Design review of the part built by this model. Coordinates are the model's own, in mm. Give positions to 0.01 mm unless a question says otherwise; leave off trailing zeros. Write each loop counter-clockwise with the first axis right and the second up, starting at its lowest first coordinate (ties: lowest second). Pieces come first, ordered by that corner, then holes. Notation, with made-up numbers: M 60,59.25 L 115,59.25 A18 cw 115,75.25 Z; hole C 79,10 d8. An arc over 180 degrees is marked long. Answer in a Markdown table with one row per item.
```python
from build123d import *

# Parameters (mm, degrees)
F0_R     = 30
F0_R_2   = 9.5
F1_DEPTH = 20
F2_DEPTH = 8
F3_D     = 5.5


with BuildPart() as f1:
    # F0 (on Front) → F1 (new body)
    with BuildSketch(Plane.XZ):
        Circle(F0_R)
        with Locations((17.2907616943, 0)):
            Circle(F0_R_2, mode=Mode.SUBTRACT)
        with Locations((17.2907616943, 0)):
            Circle(F0_R_2)
    extrude(amount=-F1_DEPTH)

    # F0 (on Front) → F2 (join)
    with BuildSketch(Plane.XZ):
        with Locations((17.2907616943, 0)):
            Circle(F0_R_2)
    extrude(amount=F2_DEPTH)

    # F3 (through all)
    with Locations(Plane.XZ):
        with Locations((0, 0)):
            Hole(F3_D / 2)


solid = f1.part
```
1) The part is to be moulded in two halves that separate along Z. For faces 1 (the face through (17, -8, 0)), 2 (the face through (7.8, -3.9, 0.4)), 3 (the face through (0.596, 10.14, -2.685)), say which applies: released by +Z, released by -Z, zero draft, split by the parting line, or undercut.
Geometry says:
| item | result |
|---|---|
| face 1 | zero draft |
| face 2 | split by the parting line |
| face 3 | undercut |
2) To check wall thickness, follow probe 1 along Z at (x, y) = (0, 6); probe 2 along Y at (x, z) = (27, 9); probe 3 along Z at (x, y) = (1.5, 5.25). State the ranges of each line that lie inside material, in increasing order. Write a range as [from, to].
Geometry says:
| item | result |
|---|---|
| probe 1 | [-30, -2.75], [2.75, 30] |
| probe 2 | [0, 20] |
| probe 3 | [-29.96, -2.3], [2.3, 29.96] |
3) Insertion check: P1, Ø6, axis at y = 4, z = 8.5, coming from the -X side; P2, Ø4.5, axis at x = 0, z = 0, coming from the +Y side; P3, Ø2, axis at x = -13.5, y = 7, coming from the -Z side; P4, Ø5, axis at x = -24, y = 10, coming from the +Z side. Each pin has a flat end and moves straight along its axis. Give the tip position at first contact, or say it passes through.
Geometry says:
| item | result |
|---|---|
| P1 | x = -29.49 |
| P2 | through |
| P3 | z = -27.27 |
| P4 | z = 20.92 |
4) Add section A-A (x = 0). Write out the cut boundary in (y, z).
Geometry says:
| item | result |
|---|---|
| outline | M 0,-30 L 20,-30 L 20,-2.75 L 0,-2.75 Z; M 0,2.75 L 20,2.75 L 20,30 L 0,30 Z |
5) Add section D-D (z = 24). Write out the cut boundary in (x, y), and give its area (3 significant figures).
Geometry says:
| item | result |
|---|---|
| outline | M -18,0 L 18,0 L 18,20 L -18,20 Z |
| area | 720 mm^2 |
6) Add section C-C (y = 2). Write out the cut boundary in (x, z), and give its area (3 significant figures).
Geometry says:
| item | result |
|---|---|
| outline | C 0,0 d60; hole C 0,0 d5.5 |
| area | 2,800 mm^2 |
7) Add section B-B (z = 0). Write out the cut boundary in (x, y), and give its area (3 significant figures).
Geometry says:
| item | result |
|---|---|
| outline | M -30,0 L -2.75,0 L -2.75,20 L -30,20 Z; M 2.75,0 L 7.79,0 L 7.79,-8 L 26.79,-8 L 26.79,0 L 30,0 L 30,20 L 2.75,20 Z |
| area | 1,240 mm^2 |
